Autodesk Inventor part; units mm, degrees
ref_plane "YZ Plane" through (0, 0, 0) normal (1, 0, 0) x (0, 1, 0)
ref_plane "XZ Plane" through (0, 0, 0) normal (0, 1, 0) x (-1, 0, 0)
ref_plane "XY Plane" through (0, 0, 0) normal (0, 0, 1) x (1, 0, 0)
sketch "Sketch1" plane through (0, 0, 0) normal (0, 0, 1) x (1, 0, 0)
  line L0 (0, 0) -> (63.5, 0)
  line L1 (63.5, 0) -> (63.5, 50.8)
  line L2 (63.5, 50.8) -> (0, 50.8)
  line L3 (0, 50.8) -> (0, 0)
  dimension "d0" = 50.8
  dimension "d1" = 63.5
extrude "Extrusion1" add sketch "Sketch1" along normal blind 1.27
sketch "Sketch2" plane through (0, 0, 1.27) normal (0, 0, 1) x (1, 0, 0)
  line L0 (63.5, 0) -> (63.5, 50.8)
  line L1 (0, 0) -> (63.5, 0)
  line L2 (63.5, 0) -> (63.5, 2.54)
  line L3 (63.5, 2.54) -> (0, 2.54)
  line L4 (0, 2.54) -> (0, 0)
  dimension "d4" = 2.54
extrude "Extrusion2" add sketch "Sketch2" along normal blind 6.35
sketch "Sketch3" plane through (0, 0, 1.27) normal (0, 0, 1) x (1, 0, 0)
  line L0 (63.5, 50.8) -> (0, 50.8)
  line L1 (63.5, 2.54) -> (63.5, 50.8)
  point P0 (0, 0)
  point P1 (31.75, 33.02)
  dimension "d7" = 17.78
  dimension "d8" = 31.75
hole "Hole1" at (31.75, 33.02, 1.27) direction (0, 0, -1) diameter 3.175 depth 25.4 tip angle 118
sketch "Sketch4" plane through (0, 0, 1.27) normal (0, 0, 1) x (1, 0, 0)
  line L0 (0, 50.8) -> (0, 2.54)
  line L1 (63.5, 2.54) -> (63.5, 50.8)
  line L2 (63.5, 50.8) -> (0, 50.8)
  point P0 (0, 0)
  point P1 (5.08, 45.72)
  point P2 (58.42, 45.72)
  dimension "d16" = 5.08
  dimension "d17" = 5.08
  dimension "d18" = 5.08
  dimension "d19" = 5.08
hole "Hole2" at (5.08, 45.72, 1.27) at (58.42, 45.72, 1.27) direction (0, 0, -1) diameter 3.1852 depth 25.4 tip angle 118
sketch "Sketch5" plane through (0, 2.54, 1.27) normal (0, 1, 0) x (1, 0, 0)
  line L0 (63.5, -6.35) -> (0, -6.35)
  line L1 (0, 0) -> (0, -6.35)
  line L2 (63.5, 0) -> (63.5, -6.35)
  point P0 (0, 1.27)
  point P1 (5.08, -3.175)
  point P2 (58.42, -3.175)
  dimension "d27" = 3.175
  dimension "d28" = 5.08
  dimension "d29" = 3.175
  dimension "d30" = 5.08
hole "Hole3" at (5.08, 2.54, 4.445) at (58.42, 2.54, 4.445) direction (0, -1, 0) diameter 3.1852 depth 25.4 tip angle 118
sketch "Sketch6" plane through (0, 0, 1.27) normal (0, 0, 1) x (1, 0, 0)
  circle A0 centre (31.75, 33.02) radius 1.5875 construction
  circle A1 centre (31.75, 33.02) radius 3.81 construction
  circle A2 centre (27.2994, 26.8348) radius 3.81 construction
  line L0 (0, 0) -> (63.5, 0)
  circle A3 centre (20.32, 30.48) radius 4.064
  circle A4 centre (27.2994, 26.8348) radius 1.5875
  circle A5 centre (5.08, 45.72) radius 1.5926
  line L1 (0, 50.8) -> (0, 2.54)
  dimension "d38" = 7.62
  dimension "d39" = 7.62
  dimension "d42" = 8.128
  dimension "d43" = 3.175
  dimension "d46" = 15.24
  dimension "d47" = 15.24
  dimension "d48" = 26.8348
  dimension "d49" = 27.2994
extrude "Extrusion3" cut sketch "Sketch6" against normal blind 25.4 contours A3 | A4
properties part number "000110-2"
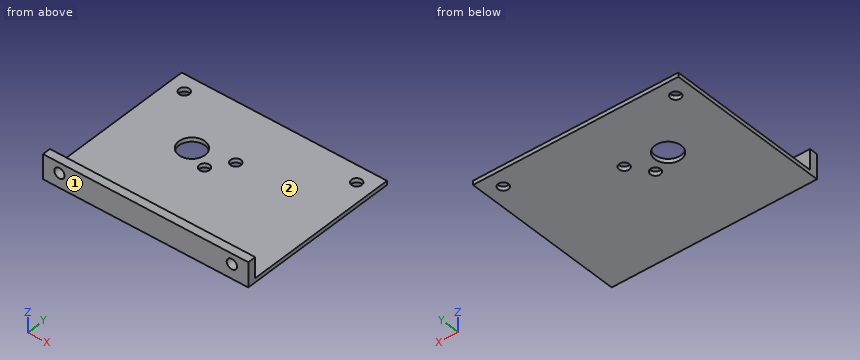
Input: part model. Units: mm. Frame: model coordinates. Face numbers are marked on the shaded views. Coordinates: 2 decimals unless noted, no trailing zeros. Loops run counter-clockwise (first coordinate to the right, second up) from the corner with the lowest first, then second, coordinate; pieces in that order, holes last. Notation, with made-up numbers: (-27, -21.5) -> (-6, -21.5) arc R13 ccw to (-6, -5.5) -> close; hole circle Ø3 at (68.25, 60). An arc over 180 degrees is marked (long way). Use a Markdown table: item, result.
1) Contact query for flat-ended pins moving along their axis: pin 1 (1 mm diameter, centred on x = 11, y = 30, fed in from +Z); pin 2 (4 mm diameter, centred on x = 10.5, z = 6.5, fed in from +Y). Output: stop coordinate, or through.
Results found:
| item | result |
|---|---|
| pin 1 | stops at z = 1.27 |
| pin 2 | stops at y = 2.54 |
2) Material intervals for line 1 along X through (y, z) = (45.72, 0.95); line 2 along Y through (x, z) = (31.75, 0.4); line 3 along Y through (x, z) = (5.08, 0.65), sorted ascending. Write a range as from..to.
Results found:
| item | result |
|---|---|
| line 1 | x = 0..3.49, 6.67..56.83, 60.01..63.5 |
| line 2 | y = 0..31.43, 34.61..50.8 |
| line 3 | y = 0..44.13, 47.31..50.8 |
3) Cut plane B-B (y = 45.72). Return the cut outline in (x, z), then the cut area to 3 significant figures.
Results found:
| item | result |
|---|---|
| outline | (0, 0) -> (3.49, 0) -> (3.49, 1.27) -> (0, 1.27) -> close; (6.67, 0) -> (56.83, 0) -> (56.83, 1.27) -> (6.67, 1.27) -> close; (60.01, 0) -> (63.5, 0) -> (63.5, 1.27) -> (60.01, 1.27) -> close |
| area | 72.6 mm2 |
4) Cut plane C-C (x = 58.42). Return the cut outline in (y, z), then the cut area to 3 significant figures.
Results found:
| item | result |
|---|---|
| outline | (0, 0) -> (44.13, 0) -> (44.13, 1.27) -> (2.54, 1.27) -> (2.54, 2.85) -> (0, 2.85) -> close; (0, 6.04) -> (2.54, 6.04) -> (2.54, 7.62) -> (0, 7.62) -> close; (47.31, 0) -> (50.8, 0) -> (50.8, 1.27) -> (47.31, 1.27) -> close |
| area | 68.5 mm2 |
5) Cut plane D-D (y = 30.48). Return the cut outline in (x, z), then the cut area to 3 significant figures.
Results found:
| item | result |
|---|---|
| outline | (0, 0) -> (16.26, 0) -> (16.26, 1.27) -> (0, 1.27) -> close; (24.38, 0) -> (63.5, 0) -> (63.5, 1.27) -> (24.38, 1.27) -> close |
| area | 70.3 mm2 |
6) Cut plane A-A (x = 20.32). Return the cut outline in (y, z), then the cut area to 3 significant figures.
Results found:
| item | result |
|---|---|
| outline | (0, 0) -> (26.42, 0) -> (26.42, 1.27) -> (2.54, 1.27) -> (2.54, 7.62) -> (0, 7.62) -> close; (34.54, 0) -> (50.8, 0) -> (50.8, 1.27) -> (34.54, 1.27) -> close |
| area | 70.3 mm2 |
7) Pull-direction query (Y, two-part tool) for the marked faces 1 and 2; classes: released by +Y, released by -Y, zero draft, split by the parting line, or undercut.
Results found:
| item | result |
|---|---|
| face 1 | released by -Y |
| face 2 | zero draft |
